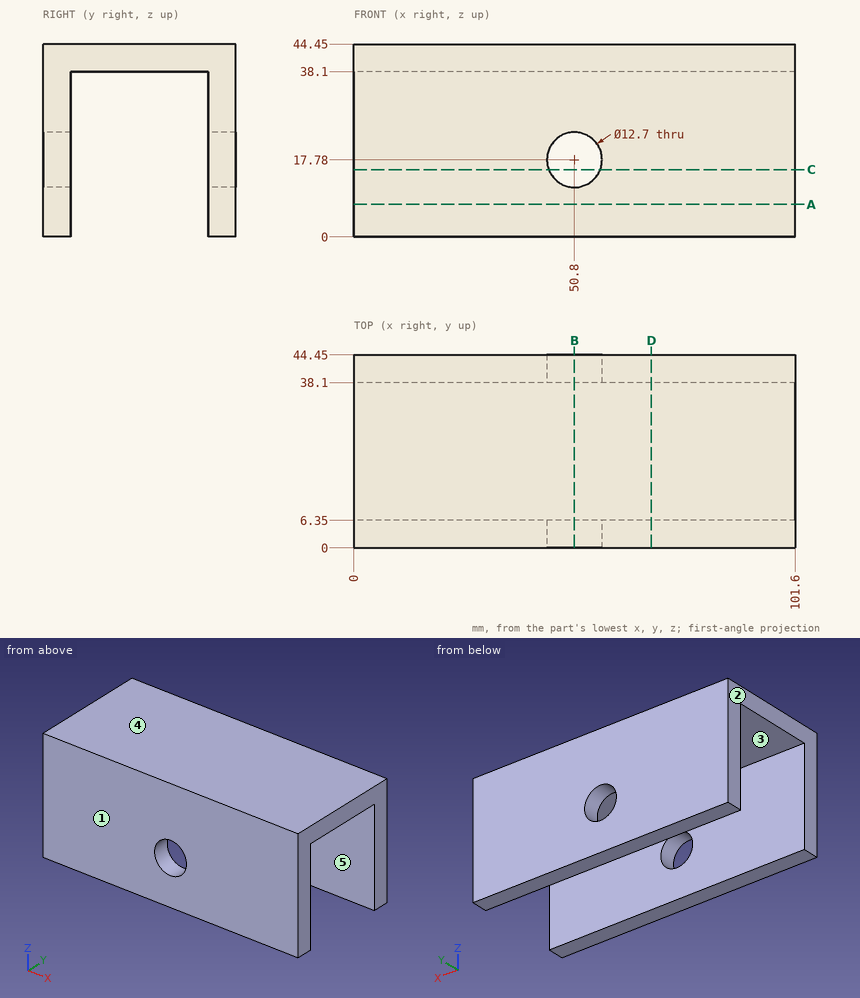
Geometry: see drawing. Coordinates: mm, zero at the bounding-box minimum. A direction names the side the tool comes from. Round coordinates to 2 decimals unless told otherwise and drop trailing zeros. Loops run counter-clockwise (first coordinate to the right, second up) from the corner with the lowest first, then second, coordinate; pieces in that order, holes last. Notation, with made-up numbers: M 57,27 L 87,27 A15 ccw 87,37 Z; hole C 10.25,-6 d11. An arc over 180 degrees is marked long. Use a Markdown table: item, result. Add a question column.
1. Cut plane D-D, the plane x = 68.5. Output: boundary loops of the cut face in (y, z), and give its area (3 significant figures).
2. Ray query, line 1 along Z through (x, y) = (50.8, 43); line 2 along Y through (x, z) = (60, 22); line 3 along X through (y, z) = (4, 17). Return the intervals inside material, ascending. Write a range as [from, to].
3. Contact query for flat-ended pins moving along their axis: pin 1 (6 mm diameter, centred on x = 77.5, y = 18, fed in from -Z); pin 2 (10 mm diameter, centred on y = 16, z = 18.5, fed in from -X); pin 3 (10 mm diameter, centred on y = 38, z = 25, fed in from -X). Output: stop coordinate, or through.
4. Cut plane A-A, the plane z = 7.5. Output: boundary loops of the cut face in (x, y).
5. Cut plane B-B, the plane x = 50.8. Output: boundary loops of the cut face in (y, z), and give its area (3 significant figures).
6. Cut plane C-C, the plane z = 15.5. Output: boundary loops of the cut face in (x, y), and give its area (3 significant figures).
7. Set-up query: the marked faces 4 and 5. Return all of +Z, -Z, +X, -X, +Y, -Y with unobstructed straight access to the full face (end or side cutting, diameter ignored); none if empty.
8. Pull-direction query (Y, two-part tool) for the marked faces 1, 2 and 3; classes: +Y half, -Y half, draft (parallel to the pull), parting line (faces both ways), or undercut.
Solution:
| question | item | result |
|---|---|---|
| 1 | outline | M 0,0 L 6.35,0 L 6.35,38.1 L 38.1,38.1 L 38.1,0 L 44.45,0 L 44.45,44.45 L 0,44.45 Z |
| 1 | area | 766 mm2 |
| 2 | line 1 | z = [0, 11.43], [24.13, 44.45] |
| 2 | line 2 | y = [0, 6.35], [38.1, 44.45] |
| 2 | line 3 | x = [0, 44.5], [57.1, 101.6] |
| 3 | pin 1 | stops at z = 38.1 |
| 3 | pin 2 | passes through |
| 3 | pin 3 | stops at x = 0 |
| 4 | outline | M 0,0 L 101.6,0 L 101.6,6.35 L 0,6.35 Z; M 0,38.1 L 101.6,38.1 L 101.6,44.45 L 0,44.45 Z |
| 5 | outline | M 0,0 L 6.35,0 L 6.35,11.43 L 0,11.43 Z; M 0,24.13 L 6.35,24.13 L 6.35,38.1 L 38.1,38.1 L 38.1,24.13 L 44.45,24.13 L 44.45,44.45 L 0,44.45 Z; M 38.1,0 L 44.45,0 L 44.45,11.43 L 38.1,11.43 Z |
| 5 | area | 605 mm2 |
| 6 | outline | M 0,0 L 44.87,0 L 44.87,6.35 L 0,6.35 Z; M 0,38.1 L 44.87,38.1 L 44.87,44.45 L 0,44.45 Z; M 56.73,0 L 101.6,0 L 101.6,6.35 L 56.73,6.35 Z; M 56.73,38.1 L 101.6,38.1 L 101.6,44.45 L 56.73,44.45 Z |
| 6 | area | 1,140 mm2 |
| 7 | face 4 | +Z, +X, -X, +Y, -Y |
| 7 | face 5 | -Z, +X, -X |
| 8 | face 1 | -Y half |
| 8 | face 2 | draft |
| 8 | face 3 | undercut |
